Input: part model. Units: mm. Frame: model coordinates. Face numbers are marked on the shaded views. A direction names the side the tool comes from. Give positions to 0.01 mm unless a question says otherwise; leave off trailing zeros. Loops run counter-clockwise (first coordinate to the right, second up) from the corner with the lowest first, then second, coordinate; pieces in that order, holes last.
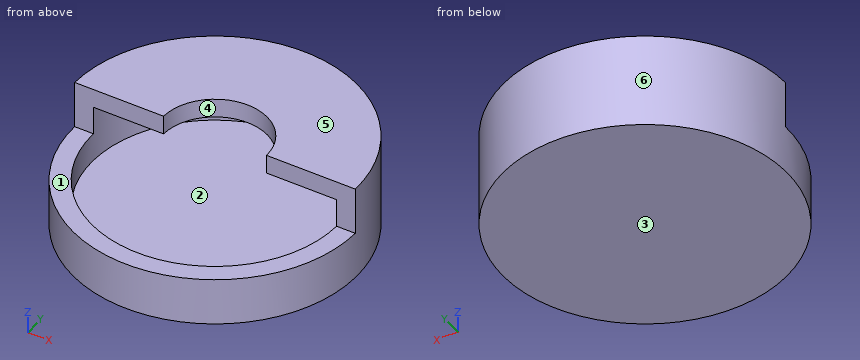
from build123d import *

# Parameters (mm, degrees)
F0_R     = 19.05
F1_DEPTH = 12.7
F3_DEPTH = 6.35
F4_T     = -2.54
F6_DEPTH = 5.08


with BuildPart() as f1:
    # F0 (on Top) → F1 (new body)
    with BuildSketch(Plane.XY):
        Circle(F0_R)
    extrude(amount=F1_DEPTH)

    # F2 (on face) → F3 (cut)
    with BuildSketch(Plane.XY.offset(12.7)):
        with BuildLine():
            ThreePointArc((19.05, 0), (0, -19.05), (-19.05, 0))
            Line((-19.05, 0), (-19.05, -19.4337088615))
            Line((-19.05, -19.4337088615), (19.2441120744, -19.4337088615))
            Line((19.2441120744, -19.4337088615), (19.2441120744, 0))
            Line((19.2441120744, 0), (19.05, 0))
        make_face()
        with BuildLine():
            Line((19.05, 0), (-19.05, 0))
            ThreePointArc((-19.05, 0), (0, -19.05), (19.05, 0))
        make_face()
    extrude(amount=-F3_DEPTH, mode=Mode.SUBTRACT)

    # F4
    f4_openings = [f1.faces().sort_by_distance(p)[0] for p in [
        (0, 0, 9.525),
        (0, -8.085071, 6.35),
    ]]
    offset(amount=F4_T, openings=f4_openings)

    # F5 (on face) → F6 (cut)
    with BuildSketch(Plane.XY.offset(12.7)):
        with BuildLine():
            Line((-6.985, 0), (6.985, 0))
            ThreePointArc((6.985, 0), (0, 6.985), (-6.985, 0))
        make_face()
    extrude(amount=-F6_DEPTH, mode=Mode.SUBTRACT)


solid = f1.part
(1) Mould query, pull axis X, two halves, no side actions, for the marked faces 4, 5 and 6. Classes: +X half, -X half, draft (parallel to the pull), parting line (faces both ways), or undercut.
Values follow:
face 4: undercut
face 5: draft
face 6: parting line
(2) Cut plane A-A (z = 4). Return the cut outline in (x, y).
Values follow:
outline: circle Ø38.1 at (0, 0); hole circle Ø33.02 at (0, 0)
(3) Ray query, probe 1 along Z at (x, y) = (-7, 14); probe 2 along Y at (x, z) = (0, 5.5); probe 3 along Z at (x, y) = (15, -6). Return the intervals inside material, ascending.
Values follow:
probe 1: z = 0 to 2.54, 10.16 to 12.7
probe 2: y = -19.05 to -16.51, 16.51 to 19.05
probe 3: z = 0 to 2.54
(4) Pin query (flat end, axial travel): pin 1 Ø5 at (x, y) = (-3.5, -8.5) entering from +Z; pin 2 Ø5 at (x, z) = (-13, 10.5) entering from -Y; pin 3 Ø2 at (y, z) = (-7.5, 6.5) entering from +X; pin 4 Ø2 at (x, y) = (-8, 1) entering from -Z. Return the tip coordinate at first contact, or that it passes through.
Values follow:
pin 1: stops at z = 2.54
pin 2: stops at y = 0
pin 3: stops at x = 17.9
pin 4: stops at z = 0
(5) Cut plane D-D (y = -8.5). Return the cut outline in (x, z), and give its area (3 significant figures).
Values follow:
outline: (-17.05, 0) - (17.05, 0) - (17.05, 6.35) - (14.15, 6.35) - (14.15, 2.54) - (-14.15, 2.54) - (-14.15, 6.35) - (-17.05, 6.35) - close
area: 109 mm2
(6) Cut plane B-B (y = 8). Return the cut outline in (x, z), and give its area (3 significant figures).
Values follow:
outline: (-17.29, 0) - (17.29, 0) - (17.29, 12.7) - (-17.29, 12.7) - close; hole (-14.44, 2.54) - (14.44, 2.54) - (14.44, 10.16) - (-14.44, 10.16) - close
area: 219 mm2
(7) Cut plane C-C (x = 0). Return the cut outline in (y, z) (3 decimals), and give its area (3 significant figures).
Values follow:
outline: (-19.05, 0) - (19.05, 0) - (19.05, 12.7) - (6.985, 12.7) - (6.985, 10.16) - (16.51, 10.16) - (16.51, 2.54) - (-16.51, 2.54) - (-16.51, 6.35) - (-19.05, 6.35) - close
area: 156 mm2
(8) Reachability of the marked faces 1, 2 and 3 from +Z, -Z, +X, -X, +Y, -Y: full face, straight path, thin tool, end or side. Return the list, or none.
Values follow:
face 1: +Z, +X, -X, -Y
face 2: none
face 3: -Z, +X, -X, +Y, -Y
